```python
from build123d import *

# Parameters (mm, degrees)
SKETCH1_R           = 2
BOSS_EXTRUDE3_DEPTH = 1.5
SKETCH5_W           = 35
SKETCH5_H           = 3
BOSS_EXTRUDE4_DEPTH = 44
BOSS_EXTRUDE5_DEPTH = 2
CUT_EXTRUDE1_DEPTH  = 67.614562972
FILLET1_R           = 2


with BuildPart() as part:
    # Sketch1 → Boss-Extrude3 (new, symmetric)
    with BuildSketch(Plane.XY):
        with BuildLine():
            Line((0, 0), (35, 0))
            Line((35, 0), (35, 20))
            ThreePointArc((35, 20), (17.5, 37.5), (0, 20))
            Line((0, 20), (0, 0))
        make_face()
        with Locations((8.249962615, 30.201823455)):
            Circle(SKETCH1_R, mode=Mode.SUBTRACT)
        with Locations((26.75, 30)):
            Circle(SKETCH1_R, mode=Mode.SUBTRACT)
        with Locations((8.25, 9.85)):
            Circle(SKETCH1_R, mode=Mode.SUBTRACT)
        with Locations((26.75, 9.85)):
            Circle(SKETCH1_R, mode=Mode.SUBTRACT)
        with BuildLine():
            Line((8.25, 23.799671038), (8.25, 16.200328962))
            ThreePointArc((8.25, 16.200328962), (17.5, 10), (26.75, 16.200328962))
            Line((26.75, 16.200328962), (26.75, 23.799671038))
            ThreePointArc((26.75, 23.799671038), (17.5, 30), (8.25, 23.799671038))
        make_face(mode=Mode.SUBTRACT)
    extrude(amount=BOSS_EXTRUDE3_DEPTH, both=True)

    # Sketch5 → Boss-Extrude4 (add)
    with BuildSketch(Plane.XY.offset(1.5)):
        with Locations((17.5, -1.5)):
            Rectangle(SKETCH5_W, SKETCH5_H)
    extrude(amount=-BOSS_EXTRUDE4_DEPTH)

    # Sketch6 → Boss-Extrude5 (add)
    with BuildSketch(Plane(origin=(35, 0, 0), x_dir=(0, 0, -1), z_dir=(1, 0, 0))):
        Polygon((1.5, 15), (1.5, 5), (6.5, 0), (16.5, 0), align=None)
    boss_extrude5 = extrude(amount=-BOSS_EXTRUDE5_DEPTH)

    # Mirror1: Boss-Extrude5 across plane
    add(boss_extrude5.mirror(Plane(origin=(17.5, 0, 0), x_dir=(0, 0, 1), z_dir=(1, 0, 0))))

    # Sketch7 → Cut-Extrude1 (cut, through all)
    with BuildSketch(Plane(origin=(0, 0, 0), x_dir=(1, 0, 0), z_dir=(0, 1, 0))):
        with BuildLine():
            Line((5, 32.5), (5, 10.5))
            ThreePointArc((5, 10.5), (7, 8.5), (9, 10.5))
            Line((9, 10.5), (9, 32.5))
            ThreePointArc((9, 32.5), (7, 34.5), (5, 32.5))
        make_face()
        with BuildLine():
            Line((26, 32.5), (26, 10.5))
            ThreePointArc((26, 10.5), (28, 8.5), (30, 10.5))
            Line((30, 10.5), (30, 32.5))
            ThreePointArc((30, 32.5), (28, 34.5), (26, 32.5))
        make_face()
        Polygon((35, 42.5), (27.17, 42.5), (35, 34.5), align=None)
        Polygon((0, 42.5), (0, 34.5), (7.83, 42.5), align=None)
    extrude(amount=-CUT_EXTRUDE1_DEPTH, mode=Mode.SUBTRACT)

    # Fillet1
    fillet1_edges = [part.edges().sort_by_distance(p)[0] for p in [
        (17.5, -3, 1.5),
        (17.5, 0, -1.5),
    ]]
    fillet(fillet1_edges, radius=FILLET1_R)


solid = part.part
```
The model under review builds one solid part; all positions refer to its coordinate system, in mm. A direction names the side the tool comes from. Give positions to 0.01 mm unless a question says otherwise; leave off trailing zeros. Write each loop counter-clockwise with the first axis right and the second up, starting at its lowest first coordinate (ties: lowest second). Pieces come first, ordered by that corner, then holes. Notation, with made-up numbers: (88, -23.75) - (131, -23.75) arc R16 cw to (131, -17.75) - close; hole circle Ø7 at (7, -16). An arc over 180 degrees is marked (long way). Answer in a Markdown table with one row per item. Add a question column.
1. Wall thickness on line 1 along Y through (x, z) = (19, -38.5); line 2 along Y through (x, z) = (26, 0); line 3 along X through (y, z) = (9, 0): over which ranges is each line inside the solid? List them lowest first. Write a range as [from, to].
2. Tool access review of faces 1 (the cylindrical face through (17.7, 30, 0)), 2 (the flat face through (2, 6, -7)), 3 (the cylindrical face through (28, -1.5, -8.5)): name each direction out of +Z, -Z, +X, -X, +Y, -Y from which nothing blocks a thin tool from reaching the whole face with its end or side.
3. We need section A-A on z = -15. Write out the cut boundary in (x, y), then the cut area to 3 significant figures.
4. Insertion check: P1, Ø4, axis at x = 12.5, z = -11, coming from the +Y side; P2, Ø3, axis at x = 23.5, y = 9.5, coming from the -Z side; P3, Ø2.5, axis at x = 8.25, y = 9.85, coming from the +Z side. Each pin has a flat end and moves straight along its axis. Give the tip position at first contact, or say it passes through.
5. We need section D-D on x = 28. Write out the cut boundary in (y, z), then the cut area to 3 significant figures.
6. Draft analysis for pull direction Y (two halves, no side actions). For faces 4 (the flat face through (34, 7.4, -9.1)), 5 (the flat face through (31.03, -1.479, -38.556)), 6 (the cylindrical face through (17.3, 10, 0)), state which applies: +Y half, -Y half, draft (parallel to the pull), parting line (faces both ways), or undercut.
7. We need section C-C on y = 3.5. Write out the cut boundary in (x, z).
8. We need section B-B on x = 17.5. Write out the cut boundary in (y, z).
Ans:
| question | item | result |
|---|---|---|
| 1 | line 1 | y = [-3, 0] |
| 1 | line 2 | y = [-2.94, 8], [11.7, 14.73], [25.27, 28.15], [31.85, 35.3] |
| 1 | line 3 | x = [0, 6.44], [10.06, 24.94], [28.56, 35] |
| 2 | face 1 | +Z, -Z |
| 2 | face 2 | -Z, +Y |
| 2 | face 3 | +Y, -Y |
| 3 | outline | (0, -3) - (5, -3) - (5, 0) - (2, 0) - (2, 1.5) - (0, 1.5) - close; (9, -3) - (26, -3) - (26, 0) - (9, 0) - close; (30, -3) - (35, -3) - (35, 1.5) - (33, 1.5) - (33, 0) - (30, 0) - close |
| 3 | area | 87.0 mm^2 |
| 4 | P1 | stops at y = 0 |
| 4 | P2 | stops at z = -1.5 |
| 4 | P3 | passes through |
| 5 | outline | (-3, -41.65) - (0, -41.65) - (0, -34.5) - (-3, -34.5) - close; (-3, -8.5) - (0, -8.5) - (0, -3.5) arc R2 cw to (2, -1.5) - (8.29, -1.5) - (8.29, 1.5) - (-1, 1.5) arc R2 ccw to (-3, -0.5) - close; (11.41, -1.5) - (28.44, -1.5) - (28.44, 1.5) - (11.41, 1.5) - close; (31.56, -1.5) - (34, -1.5) - (34, 1.5) - (31.56, 1.5) - close |
| 5 | area | 135 mm^2 |
| 6 | face 4 | +Y half |
| 6 | face 5 | draft |
| 6 | face 6 | undercut |
| 7 | outline | (0, -13) - (2, -13) - (2, -3) - (0, -3) - close; (0, -1.5) - (35, -1.5) - (35, 1.5) - (0, 1.5) - close; (33, -13) - (35, -13) - (35, -3) - (33, -3) - close |
| 8 | outline | (-3, -42.5) - (0, -42.5) - (0, -3.5) arc R2 cw to (2, -1.5) - (10, -1.5) - (10, 1.5) - (-1, 1.5) arc R2 ccw to (-3, -0.5) - close; (30, -1.5) - (37.5, -1.5) - (37.5, 1.5) - (30, 1.5) - close |
